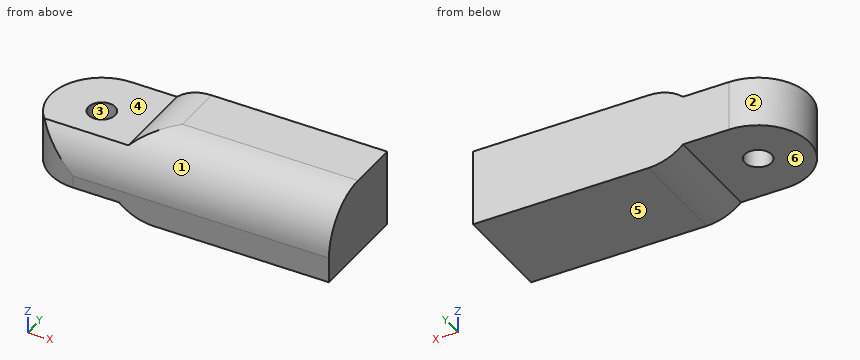
```python
from build123d import *

# Parameters (mm, degrees)
SKETCH1_R           = 2.6
BOSS_EXTRUDE1_DEPTH = 4.9
SKETCH1_3_W         = 41
SKETCH1_3_H         = 20
BOSS_EXTRUDE2_DEPTH = 7.5
FILLET1_R           = 10


with BuildPart() as part:
    # Sketch1 → Boss-Extrude1 (new, symmetric)
    with BuildSketch(Plane.XY):
        with BuildLine():
            Line((9, 10), (0, 10))
            ThreePointArc((0, 10), (-10, 0), (0, -10))
            Line((0, -10), (9, -10))
            Line((9, -10), (9, 10))
        make_face()
        Circle(SKETCH1_R, mode=Mode.SUBTRACT)
    extrude(amount=BOSS_EXTRUDE1_DEPTH, both=True)

    # Sketch1<3> → Boss-Extrude2 (add, symmetric)
    with BuildSketch(Plane.XY):
        with Locations((29.5, 0)):
            Rectangle(SKETCH1_3_W, SKETCH1_3_H)
    extrude(amount=BOSS_EXTRUDE2_DEPTH, both=True)

    # Fillet1
    # the kernel refuses this fillet: 10 mm, written as the material it takes off along each edge
    with BuildSketch(Plane(origin=(-16, -10, 7.5), x_dir=(0, 0, -1), z_dir=(1, 0, 0))) as fillet1_piece_1:
        with BuildLine():
            CenterArc((FILLET1_R, FILLET1_R), FILLET1_R, 180, 90)
            Line((0, FILLET1_R), (-FILLET1_R * 0.02, FILLET1_R))
            Line((-FILLET1_R * 0.02, FILLET1_R), (-FILLET1_R * 0.02, -FILLET1_R * 0.02))
            Line((-FILLET1_R * 0.02, -FILLET1_R * 0.02), (FILLET1_R, -FILLET1_R * 0.02))
            Line((FILLET1_R, -FILLET1_R * 0.02), (FILLET1_R, 0))
        make_face()
    extrude(amount=91, mode=Mode.SUBTRACT)
    with BuildSketch(Plane(origin=(9, 26.815171721, -7.5), x_dir=(1, 0, 0), z_dir=(0, -1, 0))) as fillet1_piece_2:
        with BuildLine():
            CenterArc((6.726068688, 10), FILLET1_R, 227.73141557, 42.26858443)
            Line((0, 2.6), (-0.134521374, 2.452))
            ThreePointArc((-0.134521374, 2.452), (-0.2, 1.3), (-0.2, 0))
            Line((-0.2, 0), (0, -0.2))
            Line((0, -0.2), (6.726068688, -0.2))
            Line((6.726068688, -0.2), (6.726068688, 0))
        make_face()
    extrude(amount=53.630343442, mode=Mode.SUBTRACT)
    with BuildSketch(Plane(origin=(9, 26.815171721, 7.5), x_dir=(1, 0, 0), z_dir=(0, -1, 0))) as fillet1_piece_3:
        with BuildLine():
            CenterArc((6.726068688, -10), FILLET1_R, 90, 42.26858443)
            Line((0, -2.6), (-0.134521374, -2.452))
            ThreePointArc((-0.134521374, -2.452), (-0.2, -1.3), (-0.2, 0))
            Line((-0.2, 0), (0, 0.2))
            Line((0, 0.2), (6.726068688, 0.2))
            Line((6.726068688, 0.2), (6.726068688, 0))
        make_face()
    extrude(amount=53.630343442, mode=Mode.SUBTRACT)


solid = part.part
```
Verification items for the finished model (mm, model axes). Face numbers are marked on the shaded views. A direction names the side the tool comes from. Round coordinates to 2 decimals unless told otherwise and drop trailing zeros. Write each loop counter-clockwise with the first axis right and the second up, starting at its lowest first coordinate (ties: lowest second). Pieces come first, ordered by that corner, then holes. Notation, with made-up numbers: (3.25, 52.25) - (37.25, 52.25) arc R31 ccw to (37.25, 77.25) - close; hole circle Ø2 at (12.5, -23). An arc over 180 degrees is marked (long way). Answer as a JSON object with one key per item and string values. Group by question number.
Q1. Tool access check on the marked faces 4, 5 and 6. Record the directions out of +Z, -Z, +X, -X, +Y, -Y that give a thin tool (end or side, any length) a straight path to the whole face; none if there is none.
Q2. Go/stop test with flat-tipped pins: pin 1 Ø6 at (y, z) = (4, -4) entering from -X; pin 2 Ø5.5 at (x, y) = (1, 0) entering from -Z. Record where each tip stops, or that it passes through.
Q3. Section check D-D, the plane x = 31. Enter the section's corners in (y, z).
Q4. Section check C-C, the plane z = 2.75. Enter the section's corners in (x, y).
Q5. Thickness scan on line 1 (Y direction, x = 0, z = 2); line 2 (Y direction, x = 0, z = 1); line 3 (Z direction, x = -4.5, y = -6.5). Record the ranges inside material, lowest first.
Q6. Section check B-B, the plane y = 8.25. Enter the section's corners in (x, z), plus the area to 3 significant figures.
Q7. Mould release check, pull along X, two halves, no side actions. Record for the marked faces 1, 2 and 3: released by +X, released by -X, zero draft, split by the parting line, or undercut.
Q8. Section check A-A, the plane x = 5. Enter the section's corners in (y, z), plus the area to 3 significant figures.
Found:
{
 "1": {"face 4": "+Z, -X, +Y, -Y", "face 5": "-Z, +X, -X, +Y, -Y", "face 6": "-Z, -X, +Y, -Y"},
 "2": {"pin 1": "stops at x = -9.95", "pin 2": "stops at z = -4.9"},
 "3": {"outline": "(-10, -7.5) - (10, -7.5) - (10, 7.5) - (0, 7.5) arc R10 ccw to (-10, -2.5) - close"},
 "4": {"outline": "(-5.25, -8.51) - (50, -8.51) - (50, 10) - (0, 10) arc R10 ccw to start; hole circle Ø5.2 at (0, 0)"},
 "5": {"line 1": "y = -8.93 to -2.6, 2.6 to 10", "line 2": "y = -9.37 to -2.6, 2.6 to 10", "line 3": "z = -4.9 to 4.9"},
 "6": {"outline": "(-5.65, -4.9) - (9, -4.9) arc R10 ccw to (15.73, -7.5) - (50, -7.5) - (50, 7.5) - (15.73, 7.5) arc R10 ccw to (9, 4.9) - (-5.65, 4.9) - close", "area": "748 mm^2"},
 "7": {"face 1": "zero draft", "face 2": "released by -X", "face 3": "undercut"},
 "8": {"outline": "(-10, -4.9) - (10, -4.9) - (10, 4.9) - (-6.73, 4.9) arc R10 ccw to (-10, -2.5) - close", "area": "189 mm^2"}
}
